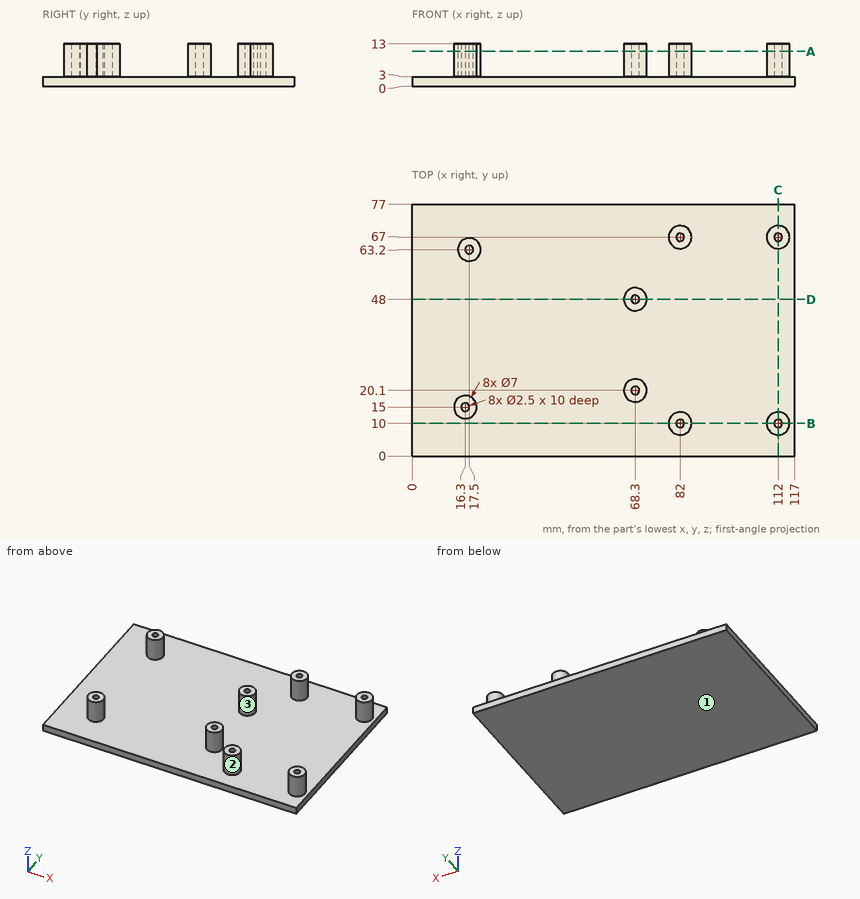
For this review, use the dimensioned drawing (mm, ordinates from the lowest corner) and the shaded views. Give positions to 0.01 mm unless a question says otherwise; leave off trailing zeros. Order: outer loops, then holes, each group sorted by start corner. A loop starts at its lowest first (then second) coordinate and runs counter-clockwise, first axis right, second up. Notation, with made-up numbers: (-21.5, -9) - (18.5, -9) arc R11 ccw to (18.5, 11) - close; hole circle Ø11 at (63, 5). An arc over 180 degrees is marked (long way). Use a Markdown table: item, result. Add a question column.
(1) Add section C-C on x = 112. Give the boundary of the cut face in (y, z).
(2) Mouldability with a two-part tool opening along X and no side actions: class the marked faces 1, 2 and 3 as +X half, -X half, draft (parallel to the pull), parting line (faces both ways), or undercut.
(3) Clearance check with a flat-ended pin moving along its axis: P1, Ø0.8, axis at x = 16.5, y = 14.5, coming from the +Z side. State where the tip first meets the part, or that it passes through.
(4) Wall thickness on probe 1 along Y at (x, z) = (68.3, 6.5); probe 2 along Y at (x, z) = (82, 10.25); probe 3 along X at (y, z) = (10.5, 5): over which ranges is each line inside the solid? List them lowest first. Write a range as [from, to].
(5) Add section D-D on y = 48. Give the boundary of the cut face in (x, z), then the cut area to 3 significant figures.
(6) Add section B-B on y = 10. Give the boundary of the cut face in (x, z), then the cut area to 3 significant figures.
(7) Add section A-A on z = 10.75. Give the number of separate pieces and of enclosed holes in the cut face, then the cut area to 3 significant figures.
Report:
| question | item | result |
|---|---|---|
| 1 | outline | (0, 0) - (77, 0) - (77, 3) - (70.5, 3) - (70.5, 13) - (68.25, 13) - (68.25, 3) - (65.75, 3) - (65.75, 13) - (63.5, 13) - (63.5, 3) - (13.5, 3) - (13.5, 13) - (11.25, 13) - (11.25, 3) - (8.75, 3) - (8.75, 13) - (6.5, 13) - (6.5, 3) - (0, 3) - close |
| 2 | face 1 | draft |
| 2 | face 2 | undercut |
| 2 | face 3 | parting line |
| 3 | P1 | stops at z = 3 |
| 4 | probe 1 | y = [16.6, 18.85], [21.35, 23.6], [44.5, 46.75], [49.25, 51.5] |
| 4 | probe 2 | y = [6.5, 8.75], [11.25, 13.5], [63.5, 65.75], [68.25, 70.5] |
| 4 | probe 3 | x = [78.54, 80.85], [83.15, 85.46], [108.54, 110.85], [113.15, 115.46] |
| 5 | outline | (0, 0) - (117, 0) - (117, 3) - (71.8, 3) - (71.8, 13) - (69.55, 13) - (69.55, 3) - (67.05, 3) - (67.05, 13) - (64.8, 13) - (64.8, 3) - (0, 3) - close |
| 5 | area | 396 mm² |
| 6 | outline | (0, 0) - (117, 0) - (117, 3) - (115.5, 3) - (115.5, 13) - (113.25, 13) - (113.25, 3) - (110.75, 3) - (110.75, 13) - (108.5, 13) - (108.5, 3) - (85.5, 3) - (85.5, 13) - (83.25, 13) - (83.25, 3) - (80.75, 3) - (80.75, 13) - (78.5, 13) - (78.5, 3) - (0, 3) - close |
| 6 | area | 441 mm² |
| 7 | separate pieces | 8 |
| 7 | enclosed holes | 8 |
| 7 | area | 269 mm² |
